Part model, mm, in its own coordinate system. A direction names the side the tool comes from. Give positions to 0.01 mm unless a question says otherwise; leave off trailing zeros. Write each loop counter-clockwise with the first axis right and the second up, starting at its lowest first coordinate (ties: lowest second). Pieces come first, ordered by that corner, then holes.
from build123d import *

# Parameters (mm, degrees)
TOP_COVER_W             = 120
TOP_COVER_H             = 25
BOSS_EXTRUDE1_DEPTH     = 3
ATTACHMENT_POINT_W      = 10.5
ATTACHMENT_POINT_H      = 15
CUT_EXTRUDE1_DEPTH      = 2
SKETCH4_R               = 1.75
M3_SCREW_CUT_DEPTH      = 62.361632964
FILLET1_R               = 2
FILLET2_R               = 2
FILLET3_R               = 2
FILLET4_R               = 2
SKETCH5_W               = 3
SKETCH5_H               = 15
CUT_EXTRUDE3_DEPTH      = 2
CONNETOR_1_ANGLE_DEPTH  = 15
CONNECTOR_2_ANGLE_DEPTH = 15


with BuildPart() as part:
    # Top Cover → Boss-Extrude1 (new body)
    with BuildSketch(Plane(origin=(0, 0, 0), x_dir=(1, 0, 0), z_dir=(0, 1, 0))):
        Rectangle(TOP_COVER_W, TOP_COVER_H)
    extrude(amount=BOSS_EXTRUDE1_DEPTH)

    # Attachment Point → Cut-Extrude1 (cut)
    with BuildSketch(Plane(origin=(0, 3, 0), x_dir=(1, 0, 0), z_dir=(0, 1, 0))):
        with Locations((-12, 0)):
            Rectangle(ATTACHMENT_POINT_W, ATTACHMENT_POINT_H)
        with Locations((12, 0)):
            Rectangle(ATTACHMENT_POINT_W, ATTACHMENT_POINT_H)
    extrude(amount=-CUT_EXTRUDE1_DEPTH, mode=Mode.SUBTRACT)

    # Sketch4 → M3 Screw CUT (cut, through all)
    with BuildSketch(Plane(origin=(0, 3, 0), x_dir=(1, 0, 0), z_dir=(0, 1, 0))):
        with Locations(Location((-12, 0, 0), (0, 0, 270))):
            Circle(SKETCH4_R)
        with Locations(Location((12, 0, 0), (0, 0, 90))):
            Circle(SKETCH4_R)
    extrude(amount=-M3_SCREW_CUT_DEPTH, mode=Mode.SUBTRACT)

    # Fillet1
    fillet1_edges = [part.edges().sort_by_distance(p)[0] for p in [
        (-60, 1.5, 12.5),
    ]]
    fillet(fillet1_edges, radius=FILLET1_R)

    # Fillet2
    fillet2_edges = [part.edges().sort_by_distance(p)[0] for p in [
        (60, 1.5, 12.5),
    ]]
    fillet(fillet2_edges, radius=FILLET2_R)

    # Fillet3
    fillet3_edges = [part.edges().sort_by_distance(p)[0] for p in [
        (60, 1.5, -12.5),
    ]]
    fillet(fillet3_edges, radius=FILLET3_R)

    # Fillet4
    fillet4_edges = [part.edges().sort_by_distance(p)[0] for p in [
        (-60, 1.5, -12.5),
    ]]
    fillet(fillet4_edges, radius=FILLET4_R)

    # Sketch5 → Cut-Extrude3 (cut)
    with BuildSketch(Plane(origin=(0, 3, 0), x_dir=(1, 0, 0), z_dir=(0, 1, 0))):
        with Locations((5.25, 0)):
            Rectangle(SKETCH5_W, SKETCH5_H)
        with Locations((-18.75, 0)):
            Rectangle(SKETCH5_W, SKETCH5_H)
    extrude(amount=-CUT_EXTRUDE3_DEPTH, mode=Mode.SUBTRACT)

    # Sketch6 → Connetor 1 Angle (add)
    with BuildSketch(Plane(origin=(0, 0, 7.5), x_dir=(-1, 0, 0), z_dir=(0, 0, -1))):
        Polygon((-4.75, 3), (-6.75, 1), (-3.75, 1), (-3.75, 3), align=None)
    extrude(amount=CONNETOR_1_ANGLE_DEPTH)

    # Sketch7 → Connector 2 Angle (add)
    with BuildSketch(Plane(origin=(0, 0, 7.5), x_dir=(-1, 0, 0), z_dir=(0, 0, -1))):
        Polygon((19.25, 3), (17.25, 1), (20.25, 1), (20.25, 3), align=None)
    extrude(amount=CONNECTOR_2_ANGLE_DEPTH)


solid = part.part
1) Flat gauge pins, fed straight in: P1, Ø3, axis at x = 12, z = 0, coming from the -Y side; P2, Ø3, axis at x = -14, z = -1, coming from the +Y side. Where does each tip first touch, or does it go through?
Check result:
P1: passes through
P2: stops at y = 1
2) Saw through at A-A (z = 0). Write the cut outline in (x, y), and give its area (3 significant figures).
Check result:
outline: (-60, 0) - (-13.75, 0) - (-13.75, 1) - (-17.25, 1) - (-19.25, 3) - (-60, 3) - close; (-10.25, 0) - (10.25, 0) - (10.25, 1) - (6.75, 1) - (4.75, 3) - (-6.75, 3) - (-6.75, 1) - (-10.25, 1) - close; (13.75, 0) - (60, 0) - (60, 3) - (17.25, 3) - (17.25, 1) - (13.75, 1) - close
area: 307 mm2
3) Drill centre lines: L1, parallel to X at y = 0.35, z = 0; L2, parallel to X at y = 2.45, z = -1; L3, parallel to Z at x = 9, y = 1.1. Where is each one in solid material? Low to high.
Check result:
L1: x = -60 to -13.75, -10.25 to 10.25, 13.75 to 60
L2: x = -60 to -18.7, -6.75 to 5.3, 17.25 to 60
L3: z = -12.5 to -7.5, 7.5 to 12.5
4) Mould opens along X. For faces 1 (the flat face through (-1, 1, -12.5)), 2 (the cylindrical face through (59.43, 1.52, -11.9)), 3 (the flat face through (-13, 2, -7.5)) say: +X half, -X half, draft (parallel to the pull), parting line (faces both ways), or undercut.
Check result:
face 1: draft
face 2: +X half
face 3: undercut
5) Saw through at C-C (y = 2.35). Write the cut outline in (x, z), and give its area (3 significant figures).
Check result:
outline: (-60, -10.5) arc R2 ccw to (-58, -12.5) - (58, -12.5) arc R2 ccw to (60, -10.5) - (60, 10.5) arc R2 ccw to (58, 12.5) - (-58, 12.5) arc R2 ccw to (-60, 10.5) - close; hole (-18.6, -7.5) - (-6.75, -7.5) - (-6.75, 7.5) - (-18.6, 7.5) - close; hole (5.4, -7.5) - (17.25, -7.5) - (17.25, 7.5) - (5.4, 7.5) - close
area: 2,640 mm2
6) Saw through at B-B (x = 12). Write the cut outline in (y, z), and give its area (3 significant figures).
Check result:
outline: (0, -12.5) - (3, -12.5) - (3, -7.5) - (1, -7.5) - (1, -1.75) - (0, -1.75) - close; (0, 1.75) - (1, 1.75) - (1, 7.5) - (3, 7.5) - (3, 12.5) - (0, 12.5) - close
area: 41.5 mm2
7) Saw through at D-D (x = -8). Write the cut outline in (y, z).
Check result:
outline: (0, -12.5) - (3, -12.5) - (3, -7.5) - (1, -7.5) - (1, 7.5) - (3, 7.5) - (3, 12.5) - (0, 12.5) - close
8) 3-axis set-ups, long thin cutter, end or side, ignore diameter. For faces 4 (the flat face through (12, 1, -2)), 5 (the flat face through (60, 1, 0)): which of +Z, -Z, +X, -X, +Y, -Y reach the whole face in a straight line?
Check result:
face 4: +Y
face 5: +Z, -Z, +X, +Y, -Y
